```python
from build123d import *

# Parameters (mm, degrees)
SKIZZE1_W                            = 20
SKIZZE1_H                            = 50
AUFSATZ_LINEAR_AUSTRAGEN1_DEPTH      = 56
SKIZZE2_R                            = 12.5
SCHNITT_LINEAR_AUSTRAGEN1_DEPTH      = 65.505813691
SKIZZE3_R                            = 1.65
SCHNITT_LINEAR_AUSTRAGEN2_DEPTH      = 15
SKIZZE4_R                            = 1.5
SCHNITT_LINEAR_AUSTRAGEN3_DEPTH      = 20
SCHNITT_LINEAR_AUSTRAGEN4_DEPTH      = 65.505813691
SCHNITT_LINEAR_AUSTRAGEN4_DEPTH_BACK = 12
SKIZZE5_R                            = 12.5
SKIZZE5_R_2                          = 3


with BuildPart() as part:
    # Skizze1 → Aufsatz-Linear austragen1 (new body)
    with BuildSketch(Plane(origin=(0, 0, 0), x_dir=(1, 0, 0), z_dir=(0, 1, 0))):
        Rectangle(SKIZZE1_W, SKIZZE1_H)
    extrude(amount=AUFSATZ_LINEAR_AUSTRAGEN1_DEPTH)

    # Skizze2 → Schnitt-Linear austragen1 (cut, through all)
    with BuildSketch(Plane.ZY.offset(10)):
        with BuildLine():
            Line((-25, 56), (-25, 31))
            ThreePointArc((-25, 31), (-17.677669509, 48.67766955), (5.8e-08, 56))
            Line((5.8e-08, 56), (-25, 56))
        make_face()
        with BuildLine():
            ThreePointArc((5.8e-08, 56), (17.67766955, 48.677669509), (25, 31))
            Line((25, 31), (25, 56))
            Line((25, 56), (5.8e-08, 56))
        make_face()
        with Locations((0, 31)):
            Circle(SKIZZE2_R)
    extrude(amount=-SCHNITT_LINEAR_AUSTRAGEN1_DEPTH, mode=Mode.SUBTRACT)

    # Skizze3 → Schnitt-Linear austragen2 (cut)
    with BuildSketch(Plane.XZ):
        with Locations(Location((0, 19, 0), (0, 0, 270))):
            Circle(SKIZZE3_R)
        with Locations(Location((0, 9, 0), (0, 0, 270))):
            Circle(SKIZZE3_R)
        with Locations(Location((0, -9, 0), (0, 0, 90))):
            Circle(SKIZZE3_R)
        with Locations(Location((0, -19, 0), (0, 0, 90))):
            Circle(SKIZZE3_R)
    extrude(amount=-SCHNITT_LINEAR_AUSTRAGEN2_DEPTH, mode=Mode.SUBTRACT)

    # Skizze4 → Schnitt-Linear austragen3 (cut)
    with BuildSketch(Plane.ZY.offset(10)):
        with Locations((-21.920310217, 31)):
            Circle(SKIZZE4_R)
        with Locations((0, 52.920310217)):
            Circle(SKIZZE4_R)
        with Locations((21.920310217, 31)):
            Circle(SKIZZE4_R)
        with Locations((0, 9.079689783)):
            Circle(SKIZZE4_R)
    extrude(amount=-SCHNITT_LINEAR_AUSTRAGEN3_DEPTH, mode=Mode.SUBTRACT)

    # Skizze5 → Schnitt-Linear austragen4 (cut, two sides: drawn at the far end of the back side and taken through both)
    with BuildSketch(Plane(origin=(10, 0, 0), x_dir=(0, 0, -1), z_dir=(1, 0, 0)).offset(-SCHNITT_LINEAR_AUSTRAGEN4_DEPTH_BACK)):
        with Locations(Location((0, 31, 0), (0, 0, 180))):
            Circle(SKIZZE5_R)
        with Locations((21.920310217, 31)):
            Circle(SKIZZE5_R_2)
        with Locations((0, 9.079689783)):
            Circle(SKIZZE5_R_2)
        with Locations((-21.920310217, 31)):
            Circle(SKIZZE5_R_2)
        with Locations((0, 52.920310217)):
            Circle(SKIZZE5_R_2)
    extrude(amount=SCHNITT_LINEAR_AUSTRAGEN4_DEPTH + SCHNITT_LINEAR_AUSTRAGEN4_DEPTH_BACK, mode=Mode.SUBTRACT)


solid = part.part
```
Geometry check sheet. Reference: the model listing, model coordinates, mm. A direction names the side the tool comes from. Round coordinates to 2 decimals unless told otherwise and drop trailing zeros. Loops run counter-clockwise (first coordinate to the right, second up) from the corner with the lowest first, then second, coordinate; pieces in that order, holes last. Notation, with made-up numbers: M 73,53 L 79,53 A25 cw 79,66 Z; hole C 71,77.25 d8. An arc over 180 degrees is marked long. Return JSON: item names as keys, results as strings. Group by question number.
(1) Section check D-D, the plane x = 7. Enter the section's corners in (y, z).
(2) Section check A-A, the plane z = -10. Enter the section's corners in (x, y), and give its area (3 significant figures).
(3) Scan lines: line 1 along X through (y, z) = (11.75, -19); line 2 along Y through (x, z) = (-4.75, -1); line 3 along Z through (x, y) = (-3.25, 9). Record each from-to range of solid material in increasing order. Write a range as [from, to].
(4) Go/stop test with flat-tipped pins: pin 1 (1.6 mm diameter, centred on x = 0.5, z = 18.5, fed in from -Y); pin 2 (2.5 mm diameter, centred on y = 52.92, z = 0, fed in from +X); pin 3 (6 mm diameter, centred on x = 1.5, y = 38, fed in from +Z); pin 4 (4.5 mm diameter, centred on x = 0, z = 9, fed in from +Y). Record where each tip stops, or that it passes through.
(5) Set-up check for faces 4 (the face through (10, 15, 0)), 5 (the face through (1, 7.4, -20.31)), 6 (the face through (3.92, 29.85, 19.15)): record each of +Z, -Z, +X, -X, +Y, -Y from which the full face is reachable in a straight line by a thin tool's end or side.
(6) Section check C-C, the plane x = 0. Enter the section's corners in (y, z).
(7) Mould release check, pull along Y, two halves, no side actions. Record for faces 1 (the face through (3.916, 31.132, -18.923)), 2 (the face through (0, 15, 25)), 3 (the face through (0, 15, 19)): pulls with the +Y half, pulls with the -Y half, needs draft (parallel to the pull), parting line crosses it, or undercut.
(8) Section check B-B, the plane y = 38.5. Enter the section's corners in (x, z).
Data:
{
 "1": {"outline": "M 0,-25 L 31,-25 A25 ccw 31,25 L 0,25 Z; hole C 9.08,0 d6; hole C 31,0 d25; hole C 31,-21.92 d6; hole C 31,21.92 d6; hole C 52.92,0 d6"},
 "2": {"outline": "M -10,0 L -1.31,0 L -1.31,15 L 1.31,15 L 1.31,0 L 10,0 L 10,23.5 L -10,23.5 Z; M -10,38.5 L 10,38.5 L 10,53.91 L -10,53.91 Z", "area": "739 mm²"},
 "3": {"line 1": "[-10, -1.65], [1.65, 10]", "line 2": "[0, 7.96], [10.2, 18.54], [43.46, 51.8], [54.04, 55.98]", "line 3": "[-25, -1.5], [1.5, 25]"},
 "4": {"pin 1": "y = 15", "pin 2": "through", "pin 3": "z = 24.68", "pin 4": "y = 55.07"},
 "5": {"face 4": "+Z, -Z, +X, +Y, -Y", "face 5": "-Y", "face 6": "+X"},
 "6": {"outline": "M 0,-25 L 31,-25 A25 ccw 31,25 L 0,25 L 0,20.65 L 15,20.65 L 15,17.35 L 0,17.35 L 0,10.65 L 15,10.65 L 15,7.35 L 0,7.35 L 0,-7.35 L 15,-7.35 L 15,-10.65 L 0,-10.65 L 0,-17.35 L 15,-17.35 L 15,-20.65 L 0,-20.65 Z; hole C 9.08,0 d6; hole C 31,0 d25; hole C 31,-21.92 d6; hole C 31,21.92 d6; hole C 52.92,0 d6"},
 "7": {"face 1": "undercut", "face 2": "needs draft", "face 3": "pulls with the -Y half"},
 "8": {"outline": "M -10,-23.85 L 10,-23.85 L 10,-10 L -10,-10 Z; M -10,10 L 10,10 L 10,23.85 L -10,23.85 Z"}
}
